Check sheet for the drawn part. Datum: minimum x, y, z corner. Units: mm. A direction names the side the tool comes from. Coordinates: 2 decimals unless noted, no trailing zeros. Order: outer loops, then holes, each group sorted by start corner. A loop starts at its lowest first (then second) coordinate and runs counter-clockwise, first axis right, second up. Notation, with made-up numbers: M -16,12.25 L -1,12.25 A12 ccw -1,18.25 Z; hole C 28,82 d2. An arc over 180 degrees is marked long. Return JSON: item names as keys, results as strings. Group by question number.
Q1. Section check D-D, the plane x = 45. Enter the section's corners in (y, z).
Q2. Thickness scan on probe 1 along X at (y, z) = (7.25, 33) (1 decimal); probe 2 along X at (y, z) = (4.75, 34) (1 decimal); probe 3 along Z at (x, y) = (13, 6.25). Record the ranges inside material, lowest first.
Q3. Access from +Z, -Z, +X, -X, +Y, -Y to the whole of each face (thin tool, end or side, straight path). Record for the marked faces 1, 2 and 3.
Q4. Section check B-B, the plane z = 9.5. Enter the section's corners in (x, y) (1 decimal), then the cut area to 3 significant figures.
Q5. Section check A-A, the plane x = 37.5. Enter the section's corners in (y, z).
Q6. Go/stop test with flat-tipped pins: pin 1 Ø3 at (x, y) = (40.5, 6) entering from -Z; pin 2 Ø1 at (x, y) = (8.5, 2.5) entering from +Z; pin 3 Ø3 at (y, z) = (6.5, 10) entering from -X. Record where each tip stops, or that it passes through.
Q7. Mould release check, pull along X, two halves, no side actions. Record for the marked faces 4, 5, 6 and 7: pulls with the +X half, pulls with the -X half, needs draft (parallel to the pull), parting line crosses it, or undercut.
Q8. Section check C-C, the plane y = 0.75. Enter the section's corners in (x, z).
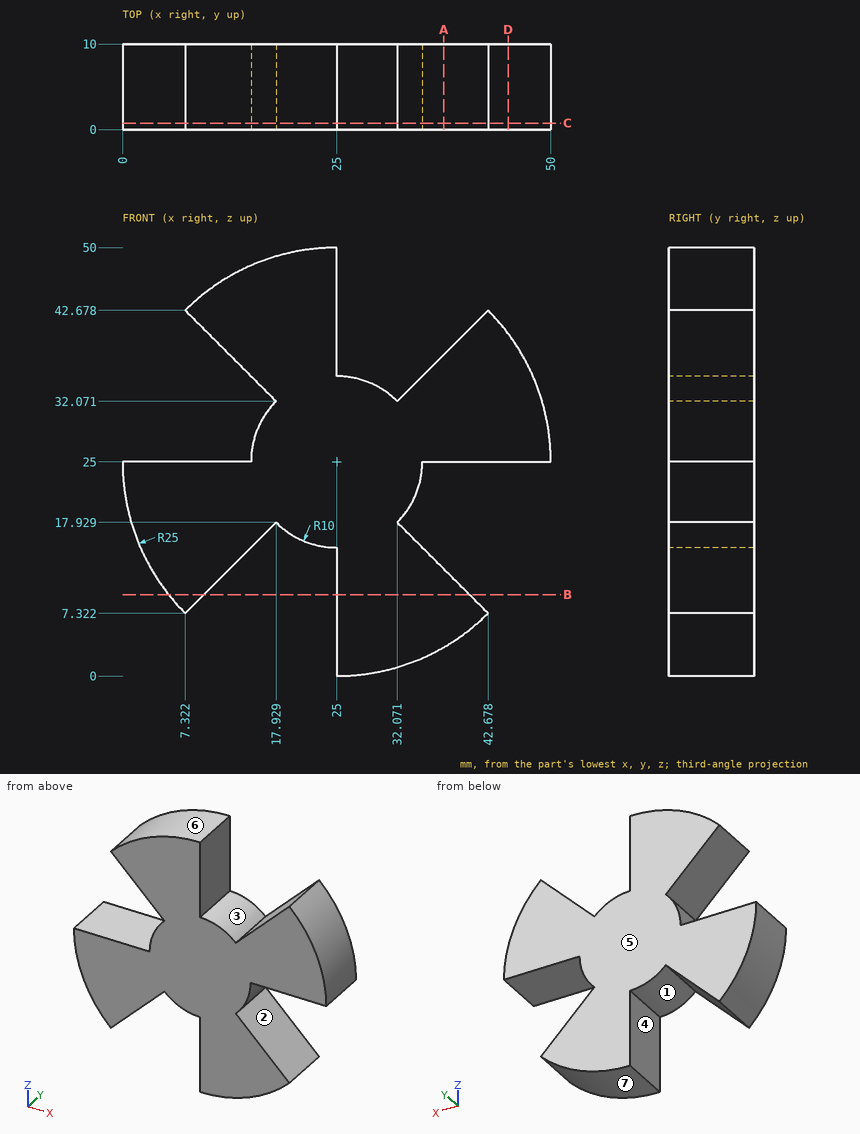
Numbers:
{
 "1": {"outline": "M 0,25 L 10,25 L 10,40 L 0,40 Z"},
 "2": {"probe 1": "x = 17 to 31, 33 to 48.7", "probe 2": "x = 16 to 29.4, 34 to 48.3", "probe 3": "z = 13 to 25, 37 to 46.93"},
 "3": {"face 1": "-Z, +Y, -Y", "face 2": "+X, +Y, -Y", "face 3": "+Z, +Y, -Y"},
 "4": {"outline": "M 5.4,0 L 9.5,0 L 9.5,10 L 5.4,10 Z; M 25,0 L 40.5,0 L 40.5,10 L 25,10 Z", "area": "196 mm2"},
 "5": {"outline": "M 0,3.35 L 10,3.35 L 10,12.5 L 0,12.5 Z; M 0,25 L 10,25 L 10,37.5 L 0,37.5 Z"},
 "6": {"pin 1": "stops at z = 4.29", "pin 2": "stops at z = 44.21", "pin 3": "stops at x = 3.96"},
 "7": {"face 4": "undercut", "face 5": "needs draft", "face 6": "pulls with the -X half", "face 7": "pulls with the +X half"},
 "8": {"outline": "M 0,25 A25 ccw 7.32,7.32 L 17.93,17.93 A10 ccw 25,15 L 25,0 A25 ccw 42.68,7.32 L 32.07,17.93 A10 ccw 35,25 L 50,25 A25 ccw 42.68,42.68 L 32.07,32.07 A10 ccw 25,35 L 25,50 A25 ccw 7.32,42.68 L 17.93,32.07 A10 ccw 15,25 Z"}
}
